from build123d import *

# Parameters (mm, degrees)
BOSS_EXTRUDE1_DEPTH = 50
SKETCH2_R           = 10
SKETCH2_R_2         = 1.5
CUT_EXTRUDE1_DEPTH  = 50


with BuildPart() as part:
    # Sketch1 → Boss-Extrude1 (new body)
    with BuildSketch(Plane.XY):
        Polygon((0, 0), (0, -60), (25.4, -60), (25.4, -57), (3, -57), (3, 0), align=None)
    extrude(amount=BOSS_EXTRUDE1_DEPTH)

    # Sketch2 → Cut-Extrude1 (cut)
    with BuildSketch(Plane(origin=(3, 0, 0), x_dir=(0, 0, -1), z_dir=(1, 0, 0))):
        with Locations((-25, -30)):
            Circle(SKETCH2_R)
        with Locations((-25, -17)):
            Circle(SKETCH2_R_2)
        with Locations((-12, -30)):
            Circle(SKETCH2_R_2)
        with Locations((-25, -43)):
            Circle(SKETCH2_R_2)
        with Locations((-38, -30)):
            Circle(SKETCH2_R_2)
    extrude(amount=-CUT_EXTRUDE1_DEPTH, mode=Mode.SUBTRACT)


solid = part.part
The model under review builds one solid part; all positions refer to its coordinate system, in mm. A direction names the side the tool comes from. Round coordinates to 2 decimals unless told otherwise and drop trailing zeros. Write each loop counter-clockwise with the first axis right and the second up, starting at its lowest first coordinate (ties: lowest second). Pieces come first, ordered by that corner, then holes. Notation, with made-up numbers: (2, 68.5) -> (14, 68.5) arc R19 cw to (14, 96.5) -> close; hole circle Ø6 at (-30.5, 44.5). An arc over 180 degrees is marked (long way). Answer as a JSON object with one key per item and string values.
1. Machinability: for faces 4 (the face through (25.4, -59, 25)), 5 (the face through (3, -29, 14)), which of the approach directions +Z, -Z, +X, -X, +Y, -Y give a long, thin tool a straight path to every point of the face, cutting with its end or side? Answer none if there is none.
Results found:
{"face 4": "+Z, -Z, +X, +Y, -Y", "face 5": "+Z, -Z, +X, +Y"}
2. We need section A-A on y = -43. State the section outline as (x, z) points.
Results found:
{"outline": "(0, 0) -> (3, 0) -> (3, 23.5) -> (0, 23.5) -> close; (0, 26.5) -> (3, 26.5) -> (3, 50) -> (0, 50) -> close"}
3. We need section D-D on z = 25. State the section outline as (x, y) points.
Results found:
{"outline": "(0, -60) -> (25.4, -60) -> (25.4, -57) -> (3, -57) -> (3, -44.5) -> (0, -44.5) -> close; (0, -41.5) -> (3, -41.5) -> (3, -40) -> (0, -40) -> close; (0, -20) -> (3, -20) -> (3, -18.5) -> (0, -18.5) -> close; (0, -15.5) -> (3, -15.5) -> (3, 0) -> (0, 0) -> close"}
4. We need section B-B on z = 12. State the section outline as (x, y) points, and give its area (3 significant figures).
Results found:
{"outline": "(0, -60) -> (25.4, -60) -> (25.4, -57) -> (3, -57) -> (3, -31.5) -> (0, -31.5) -> close; (0, -28.5) -> (3, -28.5) -> (3, 0) -> (0, 0) -> close", "area": "238 mm^2"}
5. The part is to be moulded in two halves that separate along Y. For faces 1 (the face through (0, -30, 14)), 2 (the face through (14, -57, 25)), 3 (the face through (1.521, -28.513, 12.195)), say which applies: pulls with the +Y half, pulls with the -Y half, needs draft (parallel to the pull), parting line crosses it, or undercut.
Results found:
{"face 1": "needs draft", "face 2": "pulls with the +Y half", "face 3": "undercut"}
6. To check wall thickness, follow line 1 along Y through (x, z) = (0.95, 38); line 2 along Y through (x, z) = (2.2, 25); line 3 along Y through (x, z) = (11.25, 19.5). State the ranges of each line that lie inside material, in increasing order.
Results found:
{"line 1": "y = -60 to -31.5, -28.5 to 0", "line 2": "y = -60 to -44.5, -41.5 to -40, -20 to -18.5, -15.5 to 0", "line 3": "y = -60 to -57"}
7. We need section C-C on x = 2. State the section outline as (y, z) points, and give its area (3 significant figures).
Results found:
{"outline": "(-60, 0) -> (0, 0) -> (0, 50) -> (-60, 50) -> close; hole circle Ø3 at (-43, 25); hole circle Ø20 at (-30, 25); hole circle Ø3 at (-30, 12); hole circle Ø3 at (-30, 38); hole circle Ø3 at (-17, 25)", "area": "2,660 mm^2"}
8. Clearance check with flat-ended pins moving along their axes: pin 1 (8 mm diameter, centred on x = 8.5, z = 16, fed in from +Y); pin 2 (5 mm diameter, centred on y = -7, z = 14, fed in from +X). State where each tip first meets the part, or that it passes through.
Results found:
{"pin 1": "stops at y = -57", "pin 2": "stops at x = 3"}
